Autodesk Inventor part; units mm, degrees
ref_plane "YZ Plane" through (0, 0, 0) normal (1, 0, 0) x (0, 1, 0)
ref_plane "XZ Plane" through (0, 0, 0) normal (0, 1, 0) x (-1, 0, 0)
ref_plane "XY Plane" through (0, 0, 0) normal (0, 0, 1) x (1, 0, 0)
sketch "스케치1" plane through (0, 0, 0) normal (1, 0, 0) x (0, 1, 0)
  line L0 (0, 0) -> (180, 0)
  line L1 (180, 0) -> (180, -180)
  line L2 (180, -180) -> (0, -180)
  line L3 (0, -180) -> (0, 0)
  line L4 (0, 0) -> (180, -180)
  dimension "d0" = 180
  dimension "d1" = 180
extrude "돌출1" add sketch "스케치1" along normal blind 190 contours L4 L2 L3
sketch "스케치2" plane through (0, 0, 0) normal (-1, 0, 0) x (0, 0, 1)
  line L0 (-140, 15) -> (-100, 15)
  line L1 (-100, 15) -> (-100, 35)
  line L2 (-100, 35) -> (-140, 35)
  line L3 (-140, 35) -> (-140, 15)
  line L4 (-80, 35) -> (-40, 35)
  line L5 (-40, 35) -> (-40, 15)
  line L6 (-40, 15) -> (-80, 15)
  line L7 (-80, 15) -> (-80, 35)
  line L8 (-180, 0) -> (-180, 180)
  line L9 (0, 0) -> (-180, 0)
  point P0 (-140, 25)
  point P1 (-80, 25)
  dimension "d4" = 40
  dimension "d5" = 20
  dimension "d6" = 40
  dimension "d7" = 20
  dimension "d8" = 40
  dimension "d9" = 20
  dimension "d10" = 15
  dimension "d11" = 15
  dimension "d46" = 40
extrude "돌출2" cut sketch "스케치2" against normal blind 10
sketch "스케치3" plane through (0, 15, -40) normal (0, 1, 0) x (1, 0, 0)
  line L0 (10, 0) -> (10, 40)
  line L1 (10, 0) -> (5, 0)
  line L2 (5, 0) -> (5, 40)
  line L3 (5, 40) -> (10, 40)
  line L4 (10, 40) -> (10, 0)
  line L5 (10, 100) -> (5, 100)
  line L6 (5, 100) -> (5, 60)
  line L7 (5, 60) -> (10, 60)
  line L8 (10, 60) -> (10, 100)
  point P0 (0, -40)
  dimension "d14" = 5
  dimension "d15" = 40
  dimension "d16" = 5
  dimension "d17" = 40
extrude "돌출3" cut sketch "스케치3" against normal blind 10
sketch "스케치4" plane through (190, 0, 0) normal (1, 0, 0) x (0, 0, -1)
  line L0 (140, 35) -> (100, 35)
  line L1 (100, 35) -> (100, 15)
  line L2 (100, 15) -> (140, 15)
  line L3 (140, 15) -> (140, 35)
  line L4 (80, 35) -> (40, 35)
  line L5 (40, 35) -> (40, 15)
  line L6 (40, 15) -> (80, 15)
  line L7 (80, 15) -> (80, 35)
  line L8 (180, 0) -> (180, 180)
  line L9 (0, 0) -> (180, 0)
  point P0 (140, 25)
  dimension "d20" = 40
  dimension "d21" = 20
  dimension "d22" = 40
  dimension "d23" = 20
  dimension "d24" = 20
  dimension "d25" = 40
  dimension "d26" = 15
extrude "돌출4" cut sketch "스케치4" against normal blind 10
sketch "스케치5" plane through (190, 15, -40) normal (0, 1, 0) x (1, 0, 0)
  line L0 (0, 0) -> (-10, 0)
  line L1 (-10, 0) -> (-5, 0)
  line L2 (-5, 0) -> (-5, 40)
  line L3 (-5, 40) -> (-10, 40)
  line L4 (-10, 40) -> (-10, 0)
  line L5 (-10, 60) -> (-5, 60)
  line L6 (-5, 60) -> (-5, 100)
  line L7 (-5, 100) -> (-10, 100)
  line L8 (-10, 100) -> (-10, 60)
  point P0 (-190, -40)
  dimension "d29" = 5
  dimension "d30" = 40
  dimension "d31" = 5
  dimension "d32" = 40
extrude "돌출5" cut sketch "스케치5" against normal blind 10
properties part number "ramp_3D 인쇄"
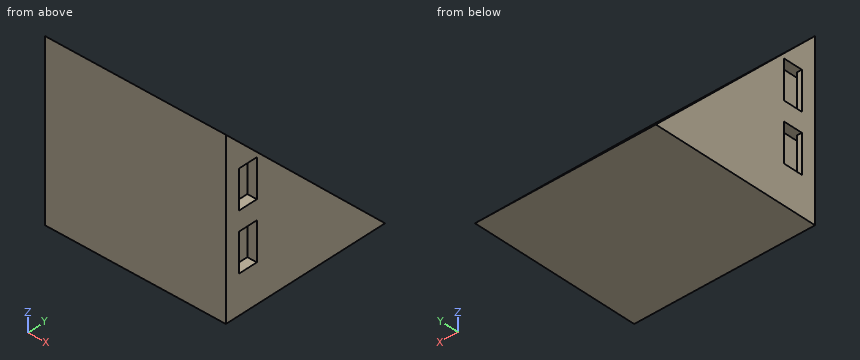
Source: CAD feature listing. Evaluate the final solid. Frame: model axes, mm. Round coordinates to 2 decimals unless told otherwise and drop trailing zeros. Loops run counter-clockwise (first coordinate to the right, second up) from the corner with the lowest first, then second, coordinate; pieces in that order, holes last.
1. Section query D-D on z = -56. Output: boundary loops of the cut face in (x, y).
2. Contact query for flat-ended pins moving along their axis: pin 1 (2 mm diameter, centred on x = 21, z = -84.5, fed in from +Y); pin 2 (4 mm diameter, centred on x = 3.5, z = -111, fed in from +Y); pin 3 (11 mm diameter, centred on x = 5, y = 19, fed in from +Z). Output: stop coordinate, or through.
3. Section query A-A on z = -126.5. Output: boundary loops of the cut face in (x, y), and give its area (3 significant figures).
4. Ray query, L1, parallel to X at y = 29, z = -123; L2, parallel to Z at x = 43, y = 63; L3, parallel to Z at x = 13.5, y = 110.5. Return the intervals inside material, ascending.
5. Section query B-B on y = 168. Output: boundary loops of the cut face in (x, z).
6. Section query C-C on x = 174. Output: boundary loops of the cut face in (y, z).
Answers below:
1. outline: (0, 0) - (190, 0) - (190, 15) - (185, 15) - (185, 5) - (180, 5) - (180, 35) - (190, 35) - (190, 56) - (0, 56) - (0, 35) - (10, 35) - (10, 5) - (5, 5) - (5, 15) - (0, 15) - close
2. pin 1: stops at y = 85.5
2. pin 2: stops at y = 113
2. pin 3: stops at z = -13.5
3. outline: (0, 0) - (190, 0) - (190, 15) - (185, 15) - (185, 5) - (180, 5) - (180, 35) - (190, 35) - (190, 126.5) - (0, 126.5) - (0, 35) - (10, 35) - (10, 5) - (5, 5) - (5, 15) - (0, 15) - close
3. area: 23,500 mm2
4. L1: x = 10 to 180
4. L2: z = -180 to -63
4. L3: z = -180 to -110.5
5. outline: (0, -180) - (190, -180) - (190, -168) - (0, -168) - close
6. outline: (0, -180) - (180, -180) - (0, 0) - close
